Could you check a few things on this model? Use its own coordinates, in mm. A direction names the side the tool comes from. Coordinates: 2 decimals unless noted, no trailing zeros. Loops run counter-clockwise (first coordinate to the right, second up) from the corner with the lowest first, then second, coordinate; pieces in that order, holes last. Notation, with made-up numbers: (45, -21) -> (68, -21) arc R32 ccw to (68, 5) -> close; hole circle Ø1 at (55.25, 33.5). An arc over 180 degrees is marked (long way). One line per question, with ' | ' between items.
Autodesk Inventor part; units mm, degrees
ref_plane "YZ Plane" through (0, 0, 0) normal (1, 0, 0) x (0, 1, 0)
ref_plane "XZ Plane" through (0, 0, 0) normal (0, 1, 0) x (-1, 0, 0)
ref_plane "XY Plane" through (0, 0, 0) normal (0, 0, 1) x (1, 0, 0)
sketch "Sketch1" plane through (0, 0, 0) normal (0, 0, 1) x (1, 0, 0)
  line L0 (-22, -11) -> (22, -11)
  line L1 (22, -11) -> (22, 11)
  line L2 (22, 11) -> (-22, 11)
  line L3 (-22, 11) -> (-22, -11)
  line L4 (-22, -11) -> (22, 11) construction
  line L5 (22, -11) -> (-22, 11) construction
  point P0 (0, 0)
  dimension "d154" = 44
  dimension "d155" = 22
extrude "Plate5" add sketch "Sketch1" along normal blind 2
fillet "Corner Round1" radius 2 2 edges at (22, 11, 1) (22, -11, 1)
sketch "Sketch10" plane through (-23.4142, 11, 3.4142) normal (0.7071068, 0, -0.7071068) x (0, 1, 0)
  line L0 (-22, 0) -> (0, 0)
  line L1 (0, 0) -> (0, -32)
  line L2 (0, -32) -> (-22, -32)
  line L3 (-22, -32) -> (-22, 0)
edge flange "Flange4" height 30 angle 45 thickness 2 bend radius 2.75 thickness toward (0.7071068, 0, -0.7071068) relief round relief width 2 relief depth 1 edges at (-22, 0, 0) wall of the first edge with corners at (-23.4142, -11, 3.4142) (-23.4142, 11, 3.4142) (-46.0416, 11, -19.2132) (-46.0416, -11, -19.2132)
bend "Bend4"
corner "Corner4"
sketch "Sketch11" plane through (-44.6274, -11, -20.6274) normal (0.7071068, 0, -0.7071068) x (-0.7071068, 0, -0.7071068)
  line L0 (-28.0325, 22) -> (-28.0325, 0) construction
  line L1 (0, 0) -> (-28.0325, 0) construction
  line L2 (0, 0) -> (0, 22) construction
  line L3 (0, 22) -> (-28.0325, 22) construction
  circle A0 centre (-10, 11) radius 5.5
  point P0 (-46.1421, 11)
  point P1 (0, 11)
  dimension "d192" = 11
  dimension "d193" = 10
extrude "Cut3" cut sketch "Sketch11" against normal blind 2
fillet "Corner Round3" radius 6 2 edges at (-45.3345, 11, -19.9203) (-45.3345, -11, -19.9203)
properties part number "TKS 3563 FDS support cup" material "Stainless Steel"
Q1. For faces 1 (the face through (0, 0, 0)), 2 (the face through (-34.07, 0.15, -7.24)), which set-ups out of +Z, -Z, +X, -X, +Y, -Y let a thin tool reach every point of the face, with its end or its side?
Values follow:
face 1: -Z, +X, +Y, -Y | face 2: +Z, -X, +Y, -Y
Q2. For pin 1 (3 mm diameter, centred on x = -5.5, y = -4.5, fed in from -Z); pin 2 (6 mm diameter, centred on y = -1.5, z = -11.5, fed in from +X); pin 3 (2 mm diameter, centred on x = -33, y = -1.5, fed in from -Z), each with a flat end and sliding along its axis, tell me the tip position at first contact or that it passes through.
Values follow:
pin 1: stops at z = 0 | pin 2: stops at x = -32.5 | pin 3: stops at z = -9.91
Q3. Imagine slicing it at A-A on y = -3.5. Write out the boundary of the cut face in (x, z), plus the area to 3 significant figures.
Values follow:
outline: (-46.04, -19.21) -> (-44.63, -20.63) -> (-40.56, -16.56) -> (-41.97, -15.14) -> close; (-35.97, -9.14) -> (-34.56, -10.56) -> (-24.81, -0.81) arc R2.75 cw to (-22.86, 0) -> (22, 0) -> (22, 2) -> (-22.86, 2) arc R4.75 ccw to (-26.22, 0.61) -> close | area: 135 mm2
Q4. Please list where these lines run through material, in increasing order: L1, parallel to Z at x = 8.5, y = 2.25; L2, parallel to X at y = 9, z = -18.5; L3, parallel to X at y = 7, z = -6.25. Write a range as [from, to].
Values follow:
L1: z = [0, 2] | L2: x = [-44.59, -42.5] | L3: x = [-33.08, -30.25]
Q5. Imagine slicing it at B-B on y = 6.5. Write out the boundary of the cut face in (x, z).
Values follow:
outline: (-45.91, -19.08) -> (-44.49, -20.49) -> (-24.81, -0.81) arc R2.75 cw to (-22.86, 0) -> (22, 0) -> (22, 2) -> (-22.86, 2) arc R4.75 ccw to (-26.22, 0.61) -> close
Q6. Imagine slicing it at C-C on x = -9. Write out the boundary of the cut face in (y, z), plus the area to 3 significant figures.
Values follow:
outline: (-11, 0) -> (11, 0) -> (11, 2) -> (-11, 2) -> close | area: 44.0 mm2
Q7. Imagine slicing it at D-D on y = 3.75. Write out the boundary of the cut face in (x, z).
Values follow:
outline: (-46.04, -19.21) -> (-44.63, -20.63) -> (-40.4, -16.4) -> (-41.82, -14.99) -> close; (-36.13, -9.3) -> (-34.71, -10.71) -> (-24.81, -0.81) arc R2.75 cw to (-22.86, 0) -> (22, 0) -> (22, 2) -> (-22.86, 2) arc R4.75 ccw to (-26.22, 0.61) -> close
